```python
from build123d import *

# Parameters (mm, degrees)
BOSS_EXTRUDE1_DEPTH = 3


with BuildPart() as part:
    # Sketch1 → Boss-Extrude1 (new body)
    with BuildSketch(Plane(origin=(0, 0, 0), x_dir=(1, 0, 0), z_dir=(0, 1, 0))):
        Polygon((-87.356947197, -190.101323735), (-90.356947197, -190.101323735), (-90.356947197, -215.101323735), (-65.356947197, -215.101323735), (-65.356947197, -212.101323735), (-50.356947197, -212.101323735), (-50.356947197, -215.101323735), (-40.356947197, -215.101323735), (-40.356947197, -212.101323735), (-25.356947197, -212.101323735), (-25.356947197, -215.101323735), (-15.356947197, -215.101323735), (-15.356947197, -212.101323735), (-0.356947197, -212.101323735), (-0.356947197, -215.101323735), (9.643052803, -215.101323735), (9.643052803, -212.101323735), (24.643052803, -212.101323735), (24.643052803, -215.101323735), (34.643052803, -215.101323735), (34.643052803, -212.101323735), (49.643052803, -212.101323735), (49.643052803, -215.101323735), (59.643052803, -215.101323735), (59.643052803, -212.101323735), (74.643052803, -212.101323735), (74.643052803, -215.101323735), (89.643052803, -215.101323735), (89.643052803, -190.101323735), (86.643052803, -190.101323735), (86.643052803, -175.101323735), (89.643052803, -175.101323735), (89.643052803, -165.101323735), (86.643052803, -165.101323735), (86.643052803, -150.101323735), (89.643052803, -150.101323735), (89.643052803, -140.101323735), (86.643052803, -140.101323735), (86.643052803, -125.101323735), (89.643052803, -125.101323735), (89.643052803, -115.101323735), (86.643052803, -115.101323735), (86.643052803, -100.101323735), (89.643052803, -100.101323735), (89.643052803, -90.101323735), (86.643052803, -90.101323735), (86.643052803, -75.101323735), (89.643052803, -75.101323735), (89.643052803, -65.101323735), (86.643052803, -65.101323735), (86.643052803, -50.101323735), (89.643052803, -50.101323735), (89.643052803, -40.101323735), (86.643052803, -40.101323735), (86.643052803, -25.101323735), (89.643052803, -25.101323735), (89.643052803, 4.898676265), (74.643052803, 4.898676265), (74.643052803, 1.898676265), (59.643052803, 1.898676265), (59.643052803, 4.898676265), (49.643052803, 4.898676265), (49.643052803, 1.898676265), (34.643052803, 1.898676265), (34.643052803, 4.898676265), (24.643052803, 4.898676265), (24.643052803, 1.898676265), (9.643052803, 1.898676265), (9.643052803, 4.898676265), (-0.356947197, 4.898676265), (-0.356947197, 1.898676265), (-15.356947197, 1.898676265), (-15.356947197, 4.898676265), (-25.356947197, 4.898676265), (-25.356947197, 1.898676265), (-40.356947197, 1.898676265), (-40.356947197, 4.898676265), (-50.356947197, 4.898676265), (-50.356947197, 1.898676265), (-65.356947197, 1.898676265), (-65.356947197, 4.898676265), (-90.356947197, 4.898676265), (-90.356947197, -25.101323735), (-87.356947197, -25.101323735), (-87.356947197, -40.101323735), (-90.356947197, -40.101323735), (-90.356947197, -50.101323735), (-87.356947197, -50.101323735), (-87.356947197, -65.101323735), (-90.356947197, -65.101323735), (-90.356947197, -75.101323735), (-87.356947197, -75.101323735), (-87.356947197, -90.101323735), (-90.356947197, -90.101323735), (-90.356947197, -100.101323735), (-87.356947197, -100.101323735), (-87.356947197, -115.101323735), (-90.356947197, -115.101323735), (-90.356947197, -125.101323735), (-87.356947197, -125.101323735), (-87.356947197, -140.101323735), (-90.356947197, -140.101323735), (-90.356947197, -150.101323735), (-87.356947197, -150.101323735), (-87.356947197, -165.101323735), (-90.356947197, -165.101323735), (-90.356947197, -175.101323735), (-87.356947197, -175.101323735), align=None)
    extrude(amount=BOSS_EXTRUDE1_DEPTH)


solid = part.part
```
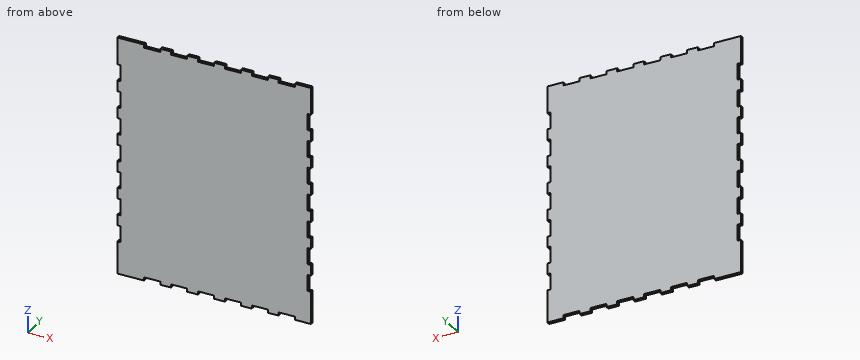
Could you check a few things on this model? Use its own coordinates, in mm. Coordinates: 2 decimals unless noted, no trailing zeros. Write each loop counter-clockwise with the first axis right and the second up, starting at its lowest first coordinate (ties: lowest second). Pieces come first, ordered by that corner, then holes. Notation, with made-up numbers: (87, 47) -> (137, 47) arc R3 cw to (137, 52) -> close; hole circle Ø4 at (43.5, 38.25). An arc over 180 degrees is marked (long way). Write item = value, one per line. Start each with the question number.
(1) I need wall thicknesses on line 1 (Z direction, x = 60.5, y = 1.7); line 2 (X direction, y = 1.6, z = 103). Which ranges of each line are inside material? Lowest first, please. Write a range as [from, to].
(2) I want a section at B-B (x = 44). Please give me the cut outline in (y, z).
(3) Will these pins go through, and if not, where does the flat tip stop? pin 1 (1 mm diameter, centred on x = -26, y = 1.5, fed in from -Z); pin 2 (1.5 mm diameter, centred on y = 1.5, z = 106.5, fed in from +X); pin 3 (10 mm diameter, centred on x = -37.5, z = 86, fed in from -Y); pin 4 (1.5 mm diameter, centred on y = 1, z = 35, fed in from -X).
(4) I want a section at A-A (z = 178.5). Please give me the cut outline in (x, y).
Result set:
q1.line_1 = [-1.9, 212.1]
q1.line_2 = [-87.36, 86.64]
q2.outline = (0, -1.9) -> (3, -1.9) -> (3, 212.1) -> (0, 212.1) -> close
q3.pin_1 = -1.9
q3.pin_2 = 86.64
q3.pin_3 = 0
q3.pin_4 = -87.36
q4.outline = (-87.36, 0) -> (86.64, 0) -> (86.64, 3) -> (-87.36, 3) -> close
